Can you work these out from the drawing? Everything is in mm from the part's minimum corner. A direction names the side the tool comes from. Coordinates: 2 decimals unless noted, no trailing zeros. Order: outer loops, then holes, each group sorted by start corner. A loop starts at its lowest first (then second) coordinate and runs counter-clockwise, first axis right, second up. Notation, with made-up numbers: (87, -5.75) -> (126, -5.75) arc R12 cw to (126, 14.25) -> close; hole circle Ø8 at (8.5, 81). An arc over 180 degrees is marked (long way). Put each result on its own line as item: value. Start each with the question number.
Q1. Will these pins go through, and if not, where does the flat tip stop? pin 1 (2 mm diameter, centred on x = 12, z = 10.5, fed in from -Y); pin 2 (2.5 mm diameter, centred on x = 14.5, y = 8.5, fed in from +Z).
Q2. If we section it at A-A (z = 7.3): Please give me the cut outline in (x, y).
Q3. If we section it at B-B (x = 17.55): Please give me the cut outline in (y, z), and give its area (3 significant figures).
Q4. If we section it at D-D (y = 3.25): Please give me the cut outline in (x, z).
Q5. We'd pull the mould along X, two halves only. Please class the marked faces 1, 2 and 3: +X half, -X half, draft (parallel to the pull), parting line (faces both ways), or undercut.
Q6. Please list where these lines run through material, in increasing order: line 1 along X through (y, z) = (7.25, 8.5); line 2 along Z through (x, y) = (13.25, 10.25); line 3 along Y through (x, z) = (13.5, 12.25).
Q7. For the marked faces 4, 5 and 6, which set-ups out of +Z, -Z, +X, -X, +Y, -Y let a thin tool reach every point of the face, with its end or its side?
Q8. If we section it at C-C (y = 7.5): Please give me the cut outline in (x, z).
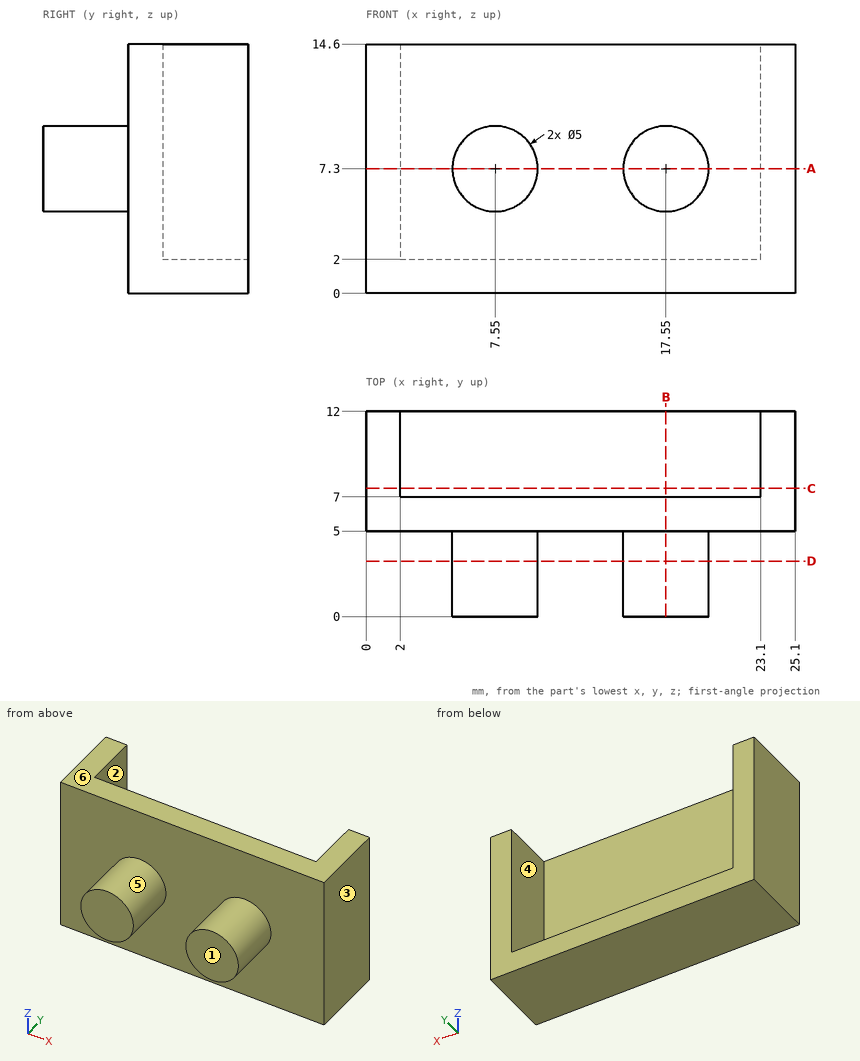
The answers:
1. pin 1: y = 5
1. pin 2: z = 2
2. outline: (0, 5) -> (5.05, 5) -> (5.05, 0) -> (10.05, 0) -> (10.05, 5) -> (15.05, 5) -> (15.05, 0) -> (20.05, 0) -> (20.05, 5) -> (25.1, 5) -> (25.1, 12) -> (23.1, 12) -> (23.1, 7) -> (2, 7) -> (2, 12) -> (0, 12) -> close
3. outline: (0, 4.8) -> (5, 4.8) -> (5, 0) -> (12, 0) -> (12, 2) -> (7, 2) -> (7, 14.6) -> (5, 14.6) -> (5, 9.8) -> (0, 9.8) -> close
3. area: 64.2 mm^2
4. outline: circle Ø5 at (7.55, 7.3); circle Ø5 at (17.55, 7.3)
5. face 1: draft
5. face 2: undercut
5. face 3: +X half
6. line 1: 0 to 2, 23.1 to 25.1
6. line 2: 0 to 2
6. line 3: 5 to 7
7. face 4: +Z, +Y
7. face 5: -Y
7. face 6: +Z, +X, -X, +Y, -Y
8. outline: (0, 0) -> (25.1, 0) -> (25.1, 14.6) -> (23.1, 14.6) -> (23.1, 2) -> (2, 2) -> (2, 14.6) -> (0, 14.6) -> close
